Input: dimensioned drawing with shaded views. Units: mm. Origin: part minimum x, y, z. A direction names the side the tool comes from. Give positions to 0.01 mm unless a question says otherwise; leave off trailing zeros. Loops run counter-clockwise (first coordinate to the right, second up) from the corner with the lowest first, then second, coordinate; pieces in that order, holes last. Notation, with made-up numbers: M -15,70.5 L 17,70.5 A20 ccw 17,75.5 Z; hole C 13,-22 d6. An arc over 180 degrees is marked long. Answer in a Markdown table with one row per item.
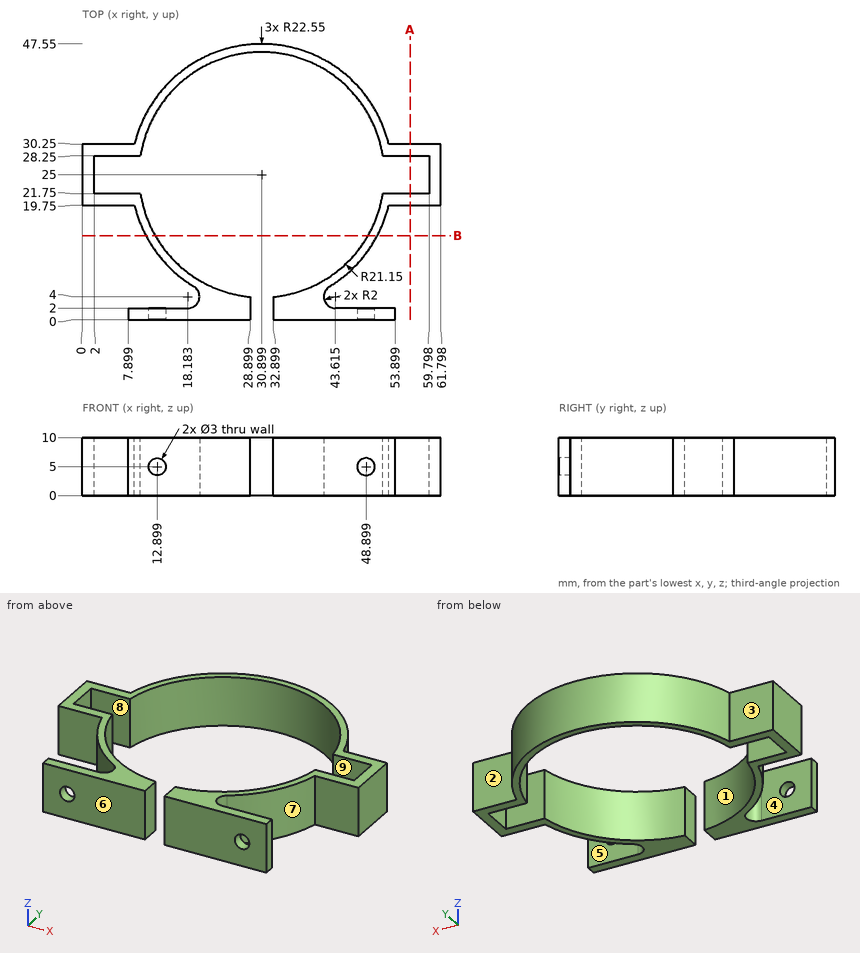
Q1. Ray query, probe 1 along Y at (x, z) = (46, 3.5) (1 decimal); probe 2 along Y at (x, z) = (4, 2); probe 3 along Y at (x, z) = (18.5, 5.5) (1 decimal). Return the intervals inside material, ascending. Write a range as from..to.
Values follow:
| item | result |
|---|---|
| probe 1 | 0..2, 8.3..10.2, 39.8..41.7 |
| probe 2 | 19.75..21.75, 28.25..30.25 |
| probe 3 | 0..2, 6.2..7.9, 42.1..43.8 |
Q2. Mould query, pull axis X, two halves, no side actions, for the marked faces 6, 7, 8 and 9. Classes: +X half, -X half, draft (parallel to the pull), parting line (faces both ways), or undercut.
Values follow:
| item | result |
|---|---|
| face 6 | draft |
| face 7 | +X half |
| face 8 | undercut |
| face 9 | undercut |
Q3. Section query A-A (x = 56.5). Output: boundary loops of the cut face in (y, z).
Values follow:
| item | result |
|---|---|
| outline | M 19.75,0 L 21.75,0 L 21.75,10 L 19.75,10 Z; M 28.25,0 L 30.25,0 L 30.25,10 L 28.25,10 Z |
Q4. Section query B-B (y = 14.5). Output: boundary loops of the cut face in (x, z) (1 decimal).
Values follow:
| item | result |
|---|---|
| outline | M 10.9,0 L 12.5,0 L 12.5,10 L 10.9,10 Z; M 49.3,0 L 50.9,0 L 50.9,10 L 49.3,10 Z |
Q5. Contact query for flat-ended pins moving along their axis: pin 1 Ø5 at (x, z) = (50.5, 3) entering from +Y; pin 2 Ø2 at (y, z) = (2.5, 3.5) entering from -X; pin 3 Ø5 at (y, z) = (37, 6) entering from +X. Output: stop coordinate, or through.
Values follow:
| item | result |
|---|---|
| pin 1 | y = 39.7 |
| pin 2 | x = 7.9 |
| pin 3 | x = 51.35 |
Q6. Reachability of the marked faces 1, 2, 3, 4 and 5 from +Z, -Z, +X, -X, +Y, -Y: full face, straight path, thin tool, end or side. Return the list, or none.
Values follow:
| item | result |
|---|---|
| face 1 | +Z, -Z |
| face 2 | +Z, -Z, +X, +Y |
| face 3 | +Z, -Z, -X, +Y |
| face 4 | +Z, -Z, -X |
| face 5 | +Z, -Z, +X |
